Autodesk Inventor part; units mm, degrees
ref_plane "YZ Plane" through (0, 0, 0) normal (1, 0, 0) x (0, 1, 0)
ref_plane "XZ Plane" through (0, 0, 0) normal (0, 1, 0) x (-1, 0, 0)
ref_plane "XY Plane" through (0, 0, 0) normal (0, 0, 1) x (1, 0, 0)
sketch "Sketch1" plane through (0, 0, 0) normal (0, 1, 0) x (-1, 0, 0)
  line L0 (-6.35, 15.24) -> (6.35, 15.24)
  line L1 (6.35, 15.24) -> (6.35, -15.24)
  line L2 (6.35, -15.24) -> (-6.35, -15.24)
  line L3 (-6.35, -15.24) -> (-6.35, 15.24)
  line L4 (-6.35, 15.24) -> (6.35, -15.24) construction
  line L5 (6.35, 15.24) -> (-6.35, -15.24) construction
  point P0 (0, 0)
  dimension "d0" = 12.7
  dimension "d1" = 30.48
extrude "Extrusion1" add sketch "Sketch1" along normal blind 12.7
sketch "Sketch2" plane through (0, 12.7, 0) normal (0, 1, 0) x (1, 0, 0)
  line L0 (-6.35, -15.24) -> (6.35, -15.24)
  line L1 (0, -15.24) -> (0, -8.89) construction
  point P0 (0, 0)
  dimension "d27" = 6.35
hole "Hole1" at (0, 12.7, 8.89) direction (0, -1, 0) diameter 6.7564 end through all
sketch "Sketch3" plane through (-6.35, 0, -15.24) normal (-1, 0, 0) x (0, 0, 1)
  line L0 (0, 0) -> (30.48, 0)
  line L1 (0, 0) -> (0, 6.35) construction
  line L2 (0, 0) -> (0, 12.7)
  line L3 (0, 6.35) -> (6.35, 6.35) construction
  point P0 (15.24, 0)
  dimension "d12" = 6.35
  dimension "d13" = 6.35
  dimension "d14" = 90
hole "Hole2" at (-6.35, 6.35, -8.89) direction (1, 0, 0) diameter 6.7564 end through all
sketch "Sketch4" plane through (-6.35, 0, -15.24) normal (-1, 0, 0) x (0, 0, 1)
  line L0 (30.48, 0) -> (30.48, 12.7)
  line L1 (30.48, 12.7) -> (12.7, 12.7)
  line L2 (12.7, 12.7) -> (12.7, 6.35)
  line L3 (12.7, 6.35) -> (30.48, 6.35)
  line L4 (30.48, 6.35) -> (30.48, 12.7)
  line L5 (0, 0) -> (0, 12.7)
  point P0 (15.24, 0)
  dimension "d23" = 6.35
  dimension "d28" = 12.7
extrude "Extrusion2" cut sketch "Sketch4" against normal up to surface (12.7 mm away)
fillet "Fillet2" radius 5.08 1 edges at (-6.35, 3.175, 15.24)
properties part number "mount" material "Aluminum 6061"
Part model, mm, in its own coordinate system. A direction names the side the tool comes from. Give positions to 0.01 mm unless a question says otherwise; leave off trailing zeros. Loops run counter-clockwise (first coordinate to the right, second up) from the corner with the lowest first, then second, coordinate; pieces in that order, holes last. Notation, with made-up numbers: M 84,41 L 109,41 A16 cw 109,66 Z; hole C 57,16.25 d11. An arc over 180 degrees is marked long. Put each result on its own line as item: value. Start each with the question number.
1) Saw through at A-A (x = 0). List the corners of the cut face in (y, z).
2) Saw through at D-D (z = 8.89). List the corners of the cut face in (x, y).
3) Saw through at B-B (x = 4.5). List the corners of the cut face in (y, z), then the cut area to 3 significant figures.
4) Saw through at C-C (y = 4.5). List the corners of the cut face in (x, z), then the cut area to 3 significant figures.
5) Flat gauge pin, fed straight in: pin 1 (3 mm diameter, centred on x = -1.5, y = 9, fed in from +Z). Where does the tip first touch, or does it go through?
6) Pull direction Z, two halves, no side cores. Call faces 3 (the flat face through (0, 10, -2.54)), 4 (the flat face through (0, 6, -15.24)), 5 (the flat face through (6.35, 5, 0)), 6 (the cylindrical face through (0.089, 5.335, -5.668)): +Z half, -Z half, draft (parallel to the pull), parting line (faces both ways), or undercut.
7) Probe probe 1 along Y at (x, z) = (-1, -8.89); probe 2 along Y at (x, z) = (-1.25, 5); probe 3 along X at (y, z) = (4, 8.89). List the from-to ranges inside material, lowest first.
8) 3-axis set-ups, long thin cutter, end or side, ignore diameter. For faces 1 (the flat face through (0, 6.35, 4)), 2 (the cylindrical face through (-4.901, 3.219, 13.712)): which of +Z, -Z, +X, -X, +Y, -Y reach the whole face in a straight line?
Numbers:
1. outline: M 0,-15.24 L 12.7,-15.24 L 12.7,-2.54 L 6.35,-2.54 L 6.35,5.51 L 0,5.51 Z; M 0,12.27 L 6.35,12.27 L 6.35,15.24 L 0,15.24 Z; hole C 6.35,-8.89 d6.76
2. outline: M -6.35,0 L -3.38,0 L -3.38,6.35 L -6.35,6.35 Z; M 3.38,0 L 6.35,0 L 6.35,6.35 L 3.38,6.35 Z
3. outline: M 0,-15.24 L 12.7,-15.24 L 12.7,-2.54 L 6.35,-2.54 L 6.35,15.24 L 0,15.24 Z; hole C 6.35,-8.89 d6.76
3. area: 238 mm^2
4. outline: M -6.35,-15.24 L 6.35,-15.24 L 6.35,-11.72 L -6.35,-11.72 Z; M -6.35,-6.06 L 6.35,-6.06 L 6.35,15.24 L -1.27,15.24 A5.08 ccw -6.35,10.16 Z; hole C 0,8.89 d6.76
4. area: 274 mm^2
5. pin 1: z = -2.54
6. face 3: +Z half
6. face 4: -Z half
6. face 5: draft
6. face 6: undercut
7. probe 1: 0 to 2.97, 9.73 to 12.7
7. probe 2: 0 to 6.35
7. probe 3: -6.35 to -3.38, 3.38 to 6.35
8. face 1: +Z, +X, -X, +Y
8. face 2: +Z, -X, +Y, -Y
